Input: part model. Units: mm. Frame: model coordinates. Give positions to 0.01 mm unless a question says otherwise; leave off trailing zeros. Order: outer loops, then holes, each group sorted by start corner. A loop starts at its lowest first (then second) coordinate and runs counter-clockwise, first axis right, second up. Notation, with made-up numbers: (43, -10.5) - (71, -10.5) arc R14 cw to (71, -2.5) - close; hole circle Ø11 at (-29, -38.75). An arc over 180 degrees is marked (long way). Use a Markdown table: item, result.
from build123d import *

# Parameters (mm, degrees)
EXTRUDE_1_DEPTH        = 535
SKETCH_2_R             = 2.5
CUT_EXTRUDE_1_DEPTH    = 1070
PATTERN_LINEAR_1_COUNT = 8
PATTERN_LINEAR_1_PITCH = 150


with BuildPart() as part:
    # Эскиз1 → Бобышка-Вытянуть1 (new, symmetric)
    with BuildSketch(Plane(origin=(0, 0, 0), x_dir=(0, 0, -1), z_dir=(1, 0, 0))):
        with BuildLine():
            Line((-6, 15), (-2.5, 18.545643943))
            ThreePointArc((-2.5, 18.545643943), (0, 30), (2.5, 18.545643943))
            Line((2.5, 18.545643943), (6, 15))
            Line((6, 15), (6, 5))
            Line((6, 5), (15, 5))
            Line((15, 5), (15, 0))
            Line((15, 0), (-15, 0))
            Line((-15, 0), (-15, 5))
            Line((-15, 5), (-6, 5))
            Line((-6, 5), (-6, 15))
        make_face()
    extrude(amount=EXTRUDE_1_DEPTH, both=True)

    # Эскиз2 → Вырез-Вытянуть1 (cut)
    with BuildSketch(Plane.XZ):
        with Locations(Location((-525, 10, 0), (0, 0, 270))):
            Circle(SKETCH_2_R)
        with Locations(Location((-525, -10, 0), (0, 0, 270))):
            Circle(SKETCH_2_R)
    cut_extrude_1 = extrude(amount=-CUT_EXTRUDE_1_DEPTH, mode=Mode.SUBTRACT)

    # Линейный массив1: Вырез-Вытянуть1 ×8
    with Locations(*[(i * PATTERN_LINEAR_1_PITCH, 0, 0) for i in range(1, PATTERN_LINEAR_1_COUNT)]):
        add(cut_extrude_1, mode=Mode.SUBTRACT)


solid = part.part
1. Material intervals for line 1 along Z through (x, y) = (375, 1); line 2 along Z through (x, y) = (-40, 6.5); line 3 along Y through (x, z) = (394.5, -3.25), sorted ascending.
Response:
| item | result |
|---|---|
| line 1 | z = -15 to -12.5, -7.5 to 7.5, 12.5 to 15 |
| line 2 | z = -6 to 6 |
| line 3 | y = 0 to 17.79, 18.96 to 29.04 |
2. Section query B-B (y = 24.5). Return loops of the section in (x, z).
Response:
| item | result |
|---|---|
| outline | (-535, -5.98) - (535, -5.98) - (535, 5.98) - (-535, 5.98) - close |
3. Section query A-A (x = 395.5). Return loops of the section in (y, z), then the cut area to 3 significant figures.
Response:
| item | result |
|---|---|
| outline | (0, -15) - (5, -15) - (5, -6) - (15, -6) - (18.55, -2.5) arc R6 ccw (long way) to (18.55, 2.5) - (15, 6) - (5, 6) - (5, 15) - (0, 15) - close |
| area | 411 mm^2 |
4. Pin query (flat end, axial travel): pin 1 (6 mm diameter, centred on x = 225, z = -10, fed in from +Y); pin 2 (6.5 mm diameter, centred on x = -375, z = -10, fed in from -Y); pin 3 (5 mm diameter, centred on x = 340.5, y = 8, fed in from -Z); pin 4 (1 mm diameter, centred on x = 272.5, y = 7.5, fed in from +Z). Return the tip coordinate at first contact, or that it passes through.
Response:
| item | result |
|---|---|
| pin 1 | stops at y = 5 |
| pin 2 | stops at y = 0 |
| pin 3 | stops at z = -6 |
| pin 4 | stops at z = 6 |
